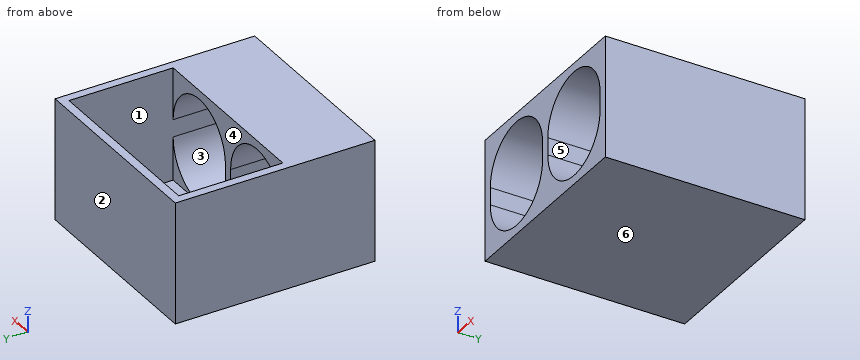
Autodesk Inventor part; units mm, degrees
ref_plane "YZ Plane" through (0, 0, 0) normal (1, 0, 0) x (0, 1, 0)
ref_plane "XZ Plane" through (0, 0, 0) normal (0, 1, 0) x (-1, 0, 0)
ref_plane "XY Plane" through (0, 0, 0) normal (0, 0, 1) x (1, 0, 0)
sketch "Base Sketch" plane through (0, 0, 0) normal (0, 0, 1) x (1, 0, 0)
  line L0 (-10.5, -6) -> (10.5, -6)
  line L1 (10.5, -6) -> (10.5, 6)
  line L2 (10.5, 6) -> (-10.5, 6)
  line L3 (-10.5, 6) -> (-10.5, -6)
  line L4 (-10.5, -6) -> (10.5, 6) construction
  line L5 (10.5, -6) -> (-10.5, 6) construction
  line L6 (-11.5, 7) -> (11.5, 7)
  line L7 (11.5, 7) -> (11.5, -16)
  line L8 (11.5, -16) -> (-11.5, -16)
  line L9 (-11.5, -16) -> (-11.5, 7)
  point P0 (0, 0)
  dimension "CavityWidth" = 21
  dimension "CavityHeight" = 12
  dimension "d5" = 1
  dimension "d6" = 1
  dimension "d7" = 1
  dimension "d8" = 10
extrude "Walls" add sketch "Base Sketch" along normal blind 14
extrude "Back" add sketch "Base Sketch" along normal blind 1 contours L3 L2 L1 L0
sketch "Whistle Hole Sketch" plane through (-10.5, -6, 14) normal (0, 1, 0) x (1, 0, 0)
  line L0 (21, 13) -> (0, 13) construction
  line L1 (0, 13) -> (0, 0) construction
  line L2 (21, 0) -> (0, 0) construction
  line L3 (21, 13) -> (21, 0) construction
  line L4 (5, 6) -> (5, 8) construction
  line L5 (10, 6) -> (10, 8)
  line L6 (0, 8) -> (0, 6)
  arc A0 (0, 6) -> (10, 6) centre (5, 6) ccw
  arc A1 (10, 8) -> (0, 8) centre (5, 8) ccw
  point P0 (10.5, 14)
  point P1 (5, 7)
  dimension "d11" = 2
  dimension "d12" = 10
extrude "Whistle Hole" cut sketch "Whistle Hole Sketch" against normal up to surface (10 mm away)
pattern_linear "Rectangular Pattern2" count 2 spacing 11 along (1, 0, 0) of "Whistle Hole"
equation "\"d5\" = WallThickness"
equation "\"d6\" = WallThickness"
equation "\"d7\" = WallThickness"
equation "\"d8\" = CapLength"
equation "\"d3\" = MaxWidth + CapOvalLength + 2 * WallThickness"
equation "\"d9\" = WallThickness"
equation "\"d20\" = WallThickness"
equation "\"d30\" = MaxWidth + SpaceBtwnKeys"
equation "\"SpaceBtwnKeys\" = 1"
equation "\"WallThickness\" = 1"
properties part number "Manifold0"
Could you check a few things on this model? Use its own coordinates, in mm. Face numbers are marked on the shaded views. A direction names the side the tool comes from. Coordinates: 2 decimals unless noted, no trailing zeros. Write each loop counter-clockwise with the first axis right and the second up, starting at its lowest first coordinate (ties: lowest second). Pieces come first, ordered by that corner, then holes. Notation, with made-up numbers: M 84.25,79.5 L 123.25,79.5 A30 cw 123.25,112.5 Z; hole C 28,-32.75 d2. An arc over 180 degrees is marked long. One line per question, with ' | ' between items.
1) For the marked faces 5 and 6, which set-ups out of +Z, -Z, +X, -X, +Y, -Y let a thin tool reach every point of the face, with its end or its side?
Checks:
face 5: -Y | face 6: -Z, +X, -X, +Y, -Y
2) If we mould it in two halves opening along Y, with no side actions, what happens to the marked faces 1, 2, 3 and 4? For each: released by +Y, released by -Y, zero draft, split by the parting line, or undercut.
Checks:
face 1: undercut | face 2: released by +Y | face 3: zero draft | face 4: undercut
3) Imagine slicing it at A-A, the plane z = 7.5. Write out the boundary of the cut face in (x, y), and give its area (3 significant figures).
Checks:
outline: M -11.5,-16 L -10.5,-16 L -10.5,6 L 10.5,6 L 10.5,-16 L 11.5,-16 L 11.5,7 L -11.5,7 Z; M -0.5,-16 L 0.5,-16 L 0.5,-6 L -0.5,-6 Z | area: 77.0 mm²
4) Imagine slicing it at C-C, the plane y = 1. Write out the boundary of the cut face in (x, z), and give its area (3 significant figures).
Checks:
outline: M -11.5,0 L 11.5,0 L 11.5,14 L 10.5,14 L 10.5,1 L -10.5,1 L -10.5,14 L -11.5,14 Z | area: 49.0 mm²
5) Imagine slicing it at D-D, the plane z = 9. Write out the boundary of the cut face in (x, y), and give its area (3 significant figures).
Checks:
outline: M -11.5,-16 L -10.4,-16 L -10.4,-6 L -10.5,-6 L -10.5,6 L 10.5,6 L 10.5,-6 L 10.4,-6 L 10.4,-16 L 11.5,-16 L 11.5,7 L -11.5,7 Z; M -0.6,-16 L 0.6,-16 L 0.6,-6 L -0.6,-6 Z | area: 81.0 mm²
6) I need wall thicknesses on probe 1 along X at (y, z) = (-14.75, 5.75); probe 2 along X at (y, z) = (-5.75, 12.75); probe 3 along Y at (x, z) = (2, 1.5). Which ranges of each line are inside material? Lowest first, please. Write a range as [from, to].
Checks:
probe 1: [-11.5, -10.49], [-0.51, 0.51], [10.49, 11.5] | probe 2: [-11.5, -10.5], [10.5, 11.5] | probe 3: [-16, -6], [6, 7]
7) Imagine slicing it at B-B, the plane x = 4. Write out the boundary of the cut face in (y, z), and give its area (3 significant figures).
Checks:
outline: M -16,0 L 7,0 L 7,14 L 6,14 L 6,1 L -6,1 L -6,1.23 L -16,1.23 Z; M -16,12.77 L -6,12.77 L -6,14 L -16,14 Z | area: 50.6 mm²
8) For pin 1 Ø3.5 at (x, y) = (-1, 0.5) entering from +Z; pin 2 Ø8 at (x, y) = (-7, -13.5) entering from -Z, each with a flat end and sliding along its axis, tell me the tip position at first contact or that it passes through.
Checks:
pin 1: z = 1 | pin 2: z = 0
